CAD build for the part. Positions are in the model's coordinates, mm. Face numbers are marked on the shaded views. A direction names the side the tool comes from. Give positions to 0.01 mm unless a question says otherwise; leave off trailing zeros. Loops run counter-clockwise (first coordinate to the right, second up) from the corner with the lowest first, then second, coordinate; pieces in that order, holes last. Notation, with made-up numbers: M 79,66.5 L 116,66.5 A32 cw 116,105.5 Z; hole C 57.25,85.25 d10. An arc over 180 degrees is marked long. Answer as CSV lines item,"result".
from build123d import *

# Parameters (mm, degrees)
F0_R     = 5
F1_DEPTH = 10
F2_R     = 2.75
F3_DEPTH = 5.001
F4_R     = 5
F5_DEPTH = 10
F6_R     = 2


with BuildPart() as f1:
    # F0 (on Front) → F1 (new body)
    with BuildSketch(Plane.XZ):
        with BuildLine():
            ThreePointArc((-0.3608562494, -8.9927627995), (-6.4902891401, -6.2350739272), (-9, 0))
            Line((-9, 0), (-14, -30))
            Line((-14, -30), (-29, -30))
            Line((-29, -30), (-29, -35))
            Line((-29, -35), (-4.6953957828, -35))
            Line((-4.6953957828, -35), (-0.3608562494, -8.9927627995))
        make_face()
        with BuildLine():
            ThreePointArc((0.3608562494, -8.9927627995), (6.4902891401, -6.2350739272), (9, 0))
            ThreePointArc((9, 0), (0, 9), (-9, 0))
            ThreePointArc((-9, 0), (-6.4902891401, -6.2350739272), (-0.3608562494, -8.9927627995))
            Line((-0.3608562494, -8.9927627995), (0, -6.827625303))
            Line((0, -6.827625303), (0.3608562494, -8.9927627995))
        make_face()
        Circle(F0_R, mode=Mode.SUBTRACT)
        with BuildLine():
            Line((14, -30), (9, 0))
            ThreePointArc((9, 0), (6.4902891401, -6.2350739272), (0.3608562494, -8.9927627995))
            Line((0.3608562494, -8.9927627995), (4.6953957828, -35))
            Line((4.6953957828, -35), (29, -35))
            Line((29, -35), (29, -30))
            Line((29, -30), (14, -30))
        make_face()
    extrude(amount=F1_DEPTH)

    # F2 (on face) → F3 (cut, through all)
    with BuildSketch(Plane.XY.offset(-30)):
        with Locations((-21.5, -5)):
            Circle(F2_R)
        with Locations((21.5, -5)):
            Circle(F2_R)
    extrude(amount=-F3_DEPTH, mode=Mode.SUBTRACT)

    # F4 (on face) → F5 (join, through all)
    with BuildSketch(Plane(origin=(0, 0, 0), x_dir=(-1, 0, 0), z_dir=(0, 1, 0))):
        with BuildLine():
            ThreePointArc((9.8245808792, -4.9474852752), (10.7021116998, -2.542598113), (11, 0))
            ThreePointArc((11, 0), (-2.542598113, 10.7021116998), (-9.8245808792, -4.9474852752))
            Line((-9.8245808792, -4.9474852752), (-9, 0))
            ThreePointArc((-9, 0), (0, 9), (9, 0))
            Line((9, 0), (9.8245808792, -4.9474852752))
        make_face()
        with BuildLine():
            Line((-9, 0), (-9.8245808792, -4.9474852752))
            ThreePointArc((-9.8245808792, -4.9474852752), (-6.0614233206, -9.1792781485), (-0.6917668776, -10.9782265684))
            Line((-0.6917668776, -10.9782265684), (0, -6.827625303))
            Line((0, -6.827625303), (0.6917668776, -10.9782265684))
            ThreePointArc((0.6917668776, -10.9782265684), (6.0614233206, -9.1792781485), (9.8245808792, -4.9474852752))
            Line((9.8245808792, -4.9474852752), (9, 0))
            ThreePointArc((9, 0), (0, 9), (-9, 0))
        make_face()
        Circle(F4_R, mode=Mode.SUBTRACT)
    extrude(amount=-F5_DEPTH)

    # F6
    f6_edges = [f1.edges().sort_by_distance(p)[0] for p in [
        (0, -5, -6.827625),
        (-14, -5, -30),
        (14, -5, -30),
        (-9.824581, -5, -4.947485),
        (9.824581, -5, -4.947485),
    ]]
    fillet(f6_edges, radius=F6_R)


solid = f1.part
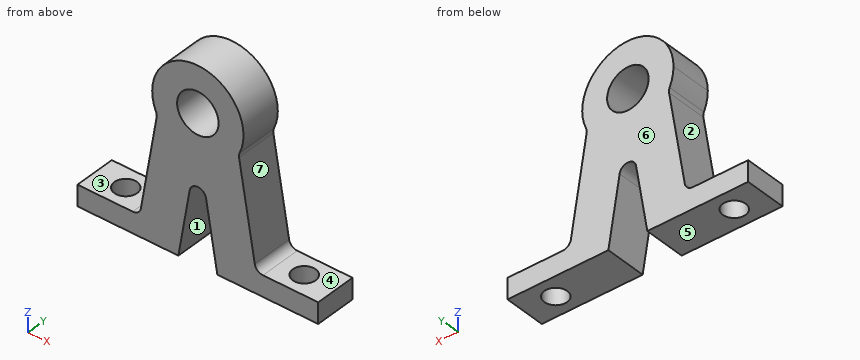
1) Band-saw the part on A-A on x = -21.5. Give the cut face in (y, z).
Answer below:
outline,"M -10,-35 L -7.75,-35 L -7.75,-30 L -10,-30 Z; M -2.25,-35 L 0,-35 L 0,-30 L -2.25,-30 Z"
2) Mould opens along Z. For the marked faces 5, 6 and 7 say: +Z half, -Z half, draft (parallel to the pull), parting line (faces both ways), or undercut.
Answer below:
face 5,"-Z half"
face 6,"draft"
face 7,"undercut"
3) Band-saw the part on B-B on y = -5. Give the number of separate pieces and of enclosed holes in the cut face, and give its area (3 significant figures).
Answer below:
separate pieces,"3"
enclosed holes,"1"
area,"936 mm^2"
4) Flat gauge pins, fed straight in: pin 1 (5 mm diameter, centred on x = -21.5, y = -5, fed in from -Z); pin 2 (6 mm diameter, centred on y = -8.5, z = -7, fed in from -X); pin 3 (2 mm diameter, centred on y = -6, z = -26, fed in from +X); pin 4 (1.5 mm diameter, centred on y = -8, z = -23.5, fed in from +X). Where does each tip first touch, or does it go through?
Answer below:
pin 1,"passes through"
pin 2,"stops at x = -10.67"
pin 3,"stops at x = 13.5"
pin 4,"stops at x = 13.04"
5) Which spindle directions (+Z, -Z, +X, -X, +Y, -Y) get a long thin tool onto all of the face, cutting with end or side? Do the marked faces 1, 2, 3 and 4. Say none if no direction does.
Answer below:
face 1,"-Z, +Y, -Y"
face 2,"-X, +Y, -Y"
face 3,"+Z, -X, +Y, -Y"
face 4,"+Z, +X, +Y, -Y"
6) Drill centre lines: line 1 (X direction, y = -4.75, z = 0); line 2 (Z direction, x = 0, y = -9); line 3 (Y direction, x = 21.5, z = -32.5). Where is each one in solid material? Low to high. Write a range as from..to.
Answer below:
line 1,"x = -11..-5, 5..11"
line 2,"z = -16.99..-5, 5..11"
line 3,"y = -10..-7.75, -2.25..0"
7) Band-saw the part on D-D on x = 12. Give the cut face in (y, z).
Answer below:
outline,"M -10,-35 L 0,-35 L 0,-18 L -10,-18 Z"
8) Band-saw the part on C-C on z = 4. Give the cut face in (x, y), and give its area (3 significant figures).
Answer below:
outline,"M -10.25,-10 L -3,-10 L -3,0 L -10.25,0 Z; M 3,-10 L 10.25,-10 L 10.25,0 L 3,0 Z"
area,"145 mm^2"
